```python
from build123d import *

# Parameters (mm, degrees)
SKETCH_1_W                   = 300
SKETCH_1_H                   = 300
EXTRUDE_1_DEPTH              = 10
SKETCH_2_W                   = 100
SKETCH_2_H                   = 100
SKETCH_2_W_2                 = 90
SKETCH_2_H_2                 = 90
EXTRUDE_2_DEPTH              = 780
SKETCH_3_R                   = 80
EXTRUDE_4_DEPTH              = 10
FILLET_3_R                   = 10
HOLE_WIZARD_M8_1_D           = 6.8
HOLE_WIZARD_M8_1_DEPTH       = 10
HOLE_WIZARD_M8_1_CSINK_D     = 8.05
HOLE_WIZARD_M8_1_CSINK_ANGLE = 90
HOLE_WIZARD_M8_1_TIP         = 2.042926105
SKETCH_7_R                   = 6.25
CUT_EXTRUDE_1_DEPTH          = 818.985329942
MIRROR_2_COPY_1_SKETCH_R     = 6.25
MIRROR_2_COPY_1_DEPTH        = 818.985329942
SKETCH_8_W                   = 10
SKETCH_8_H                   = 150
EXTRUDE_5_DEPTH              = 80
CUT_EXTRUDE_2_DEPTH          = 829.568041865
PATTERN_CIRCULAR_1_COUNT     = 4
FILLET_4_R                   = 50


with BuildPart() as part:
    # 草图1 → 凸台-拉伸1 (new body)
    with BuildSketch(Plane(origin=(0, 0, 0), x_dir=(1, 0, 0), z_dir=(0, 1, 0))):
        Rectangle(SKETCH_1_W, SKETCH_1_H)
    extrude(amount=EXTRUDE_1_DEPTH)

    # 草图2 → 凸台-拉伸2 (add)
    with BuildSketch(Plane(origin=(0, 10, 0), x_dir=(1, 0, 0), z_dir=(0, 1, 0))):
        Rectangle(SKETCH_2_W, SKETCH_2_H)
        Rectangle(SKETCH_2_W_2, SKETCH_2_H_2, mode=Mode.SUBTRACT)
    extrude(amount=EXTRUDE_2_DEPTH)

    # 草图3 → 凸台-拉伸4 (add)
    with BuildSketch(Plane(origin=(0, 790, 0), x_dir=(1, 0, 0), z_dir=(0, 1, 0))):
        with Locations(Location((0, 0, 0), (0, 0, 270))):
            Circle(SKETCH_3_R)
    extrude(amount=EXTRUDE_4_DEPTH)

    # 圆角3
    fillet_3_edges = [part.edges().sort_by_distance(p)[0] for p in [
        (50, 400, 50),
        (50, 400, -50),
        (-50, 400, -50),
        (-50, 400, 50),
        (45, 400, -45),
        (-45, 400, -45),
        (-45, 400, 45),
        (45, 400, 45),
    ]]
    fillet(fillet_3_edges, radius=FILLET_3_R)

    # M8 螺纹孔1
    with Locations(Plane(origin=(-66, 800, 0), x_dir=(0, 0, 1), z_dir=(0, 1, 0))):
        with Locations((0, 0), (-46.669047558, 19.330952442), (-66, 66), (-46.669047558, 112.669047558), (0, 132), (46.669047558, 112.669047558), (66, 66), (46.669047558, 19.330952442)):
            CounterSinkHole(HOLE_WIZARD_M8_1_D / 2, HOLE_WIZARD_M8_1_CSINK_D / 2, depth=HOLE_WIZARD_M8_1_DEPTH, counter_sink_angle=HOLE_WIZARD_M8_1_CSINK_ANGLE)
            with Locations((0, 0, -(HOLE_WIZARD_M8_1_DEPTH + HOLE_WIZARD_M8_1_TIP / 2))):  # 118° drill point
                Cone(0, HOLE_WIZARD_M8_1_D / 2, HOLE_WIZARD_M8_1_TIP, mode=Mode.SUBTRACT)

    # 草图7 → 切除-拉伸1 (cut, through all)
    with BuildSketch(Plane(origin=(0, 10, 0), x_dir=(1, 0, 0), z_dir=(0, 1, 0))):
        with Locations(Location((120, 120, 0), (0, 0, 270))):
            Circle(SKETCH_7_R)
        with Locations(Location((90, 90, 0), (0, 0, 270))):
            Circle(SKETCH_7_R)
    cut_extrude_1 = extrude(amount=-CUT_EXTRUDE_1_DEPTH, mode=Mode.SUBTRACT)

    # 镜向1: 切除-拉伸1 across plane
    add(cut_extrude_1.mirror(Plane.XY), mode=Mode.SUBTRACT)

    # 镜向2: 切除-拉伸1 across plane
    add(cut_extrude_1.mirror(Plane(origin=(0, 0, 0), x_dir=(0, 0, 1), z_dir=(1, 0, 0))), mode=Mode.SUBTRACT)

    # 镜向2 copy 1 sketch → 镜向2 copy 1 (cut, through all)
    with BuildSketch(Plane(origin=(0, 10, 0), x_dir=(-1, 0, 0), z_dir=(0, 1, 0))):
        with Locations(Location((120, 120, 0), (0, 0, 270))):
            Circle(MIRROR_2_COPY_1_SKETCH_R)
        with Locations(Location((90, 90, 0), (0, 0, 270))):
            Circle(MIRROR_2_COPY_1_SKETCH_R)
    extrude(amount=-MIRROR_2_COPY_1_DEPTH, mode=Mode.SUBTRACT)

    # 草图8 → 凸台-拉伸5 (add)
    with BuildSketch(Plane(origin=(0, 0, -50), x_dir=(-1, 0, 0), z_dir=(0, 0, -1))):
        with Locations((0, 85)):
            Rectangle(SKETCH_8_W, SKETCH_8_H)
    extrude_5 = extrude(amount=EXTRUDE_5_DEPTH)

    # 草图9 → 切除-拉伸2 (cut, through all)
    with BuildSketch(Plane(origin=(5, 0, 0), x_dir=(0, 0, -1), z_dir=(1, 0, 0))):
        Polygon((50, 160), (130, 10), (130, 160), align=None)
    cut_extrude_2 = extrude(amount=-CUT_EXTRUDE_2_DEPTH, mode=Mode.SUBTRACT)

    # 阵列(圆周)1: 凸台-拉伸5, 切除-拉伸2 ×4 about axis
    pattern_circular_1_axis = Axis((0, 0, 0), (0, 1, 0))
    add([extrude_5.rotate(pattern_circular_1_axis, i * 360 / PATTERN_CIRCULAR_1_COUNT) for i in range(1, PATTERN_CIRCULAR_1_COUNT)])
    add([cut_extrude_2.rotate(pattern_circular_1_axis, i * 360 / PATTERN_CIRCULAR_1_COUNT) for i in range(1, PATTERN_CIRCULAR_1_COUNT)], mode=Mode.SUBTRACT)

    # 圆角4
    fillet_4_edges = [part.edges().sort_by_distance(p)[0] for p in [
        (150, 5, 150),
        (-150, 5, 150),
        (-150, 5, -150),
        (150, 5, -150),
    ]]
    fillet(fillet_4_edges, radius=FILLET_4_R)


solid = part.part
```
CAD build for the part. Positions are in the model's coordinates, mm. A direction names the side the tool comes from. Coordinates: 2 decimals unless noted, no trailing zeros. Order: outer loops, then holes, each group sorted by start corner. A loop starts at its lowest first (then second) coordinate and runs counter-clockwise, first axis right, second up. Notation, with made-up numbers: (84, -20.75) -> (118, -20.75) arc R13 cw to (118, 2.25) -> close; hole circle Ø9 at (5.5, 41.25). An arc over 180 degrees is marked (long way). Use one line per item in the form item = value. Start each with the question number.
1) Drop flat-ended pins along their axis: pin 1 (8 mm diameter, centred on y = 365, z = -19, fed in from +X); pin 2 (4 mm diameter, centred on y = 571.5, z = -12.5, fed in from -X); pin 3 (16 mm diameter, centred on x = -90, z = 90, fed in from +Y); pin 4 (7.5 mm diameter, centred on x = 90, z = -90, fed in from -Y). Give the stop position or say it passes through.
2) Band-saw the part on A-A on y = 232.5. Give the cut face in (x, z), then the cut area to 3 significant figures.
3) Pull direction Y, two halves, no side cores. Call faces 1 (the cylindrical face through (-135.742, 5.07, -134.964)), 2 (the flat face through (81, 67, -5)), 3 (the flat face through (1, 800, -1)): +Y half, -Y half, draft (parallel to the pull), parting line (faces both ways), or undercut.
4) Tool access for faces 4 (the flat face through (1, 790, 52)), 5 (the flat face through (-5, 67, 81)), 6 (the cylindrical face through (-78.1, 794.93, -17.34)), 7 (the flat face through (5, 67, 81)), 8 (the flat face through (-0.07, 86.05, 89.44)): list every direction of +Z, -Z, +X, -X, +Y, -Y with a clear straight run to the whole face (end or side of a thin tool).
5) Drill centre lines: L1, parallel to X at y = 6, z = 90; L2, parallel to Y at x = -31, z = 40.5. Where is each one in solid material? Low to high. Write a range as [from, to].
Entries:
q1.pin_1 = 50
q1.pin_2 = -50
q1.pin_3 = 10
q1.pin_4 = through
q2.outline = (-50, -40) arc R10 ccw to (-40, -50) -> (40, -50) arc R10 ccw to (50, -40) -> (50, 40) arc R10 ccw to (40, 50) -> (-40, 50) arc R10 ccw to (-50, 40) -> close; hole (-45, -35) arc R10 ccw to (-35, -45) -> (35, -45) arc R10 ccw to (45, -35) -> (45, 35) arc R10 ccw to (35, 45) -> (-35, 45) arc R10 ccw to (-45, 35) -> close
q2.area = 1,900 mm2
q3.face_1 = draft
q3.face_2 = undercut
q3.face_3 = +Y half
q4.face_4 = none
q4.face_5 = +Z, -X
q4.face_6 = +Y
q4.face_7 = +Z, +X
q4.face_8 = +Z, +X, -X
q5.L1 = [-150, -96.25], [-83.75, 83.75], [96.25, 150]
q5.L2 = [0, 10], [790, 800]
